Drawing for the job (mm, zero at the part's lowest x, y, z). Coordinates: 2 decimals unless noted, no trailing zeros. Order: outer loops, then holes, each group sorted by start corner. A loop starts at its lowest first (then second) coordinate and runs counter-clockwise, first axis right, second up. Notation, with made-up numbers: (65, 86.25) - (113, 86.25) arc R8 cw to (113, 90.25) - close; hole circle Ø4 at (-20.75, 70.5). An arc over 180 degrees is marked (long way). Put each result on its own line as item: value. Start each with the question number.
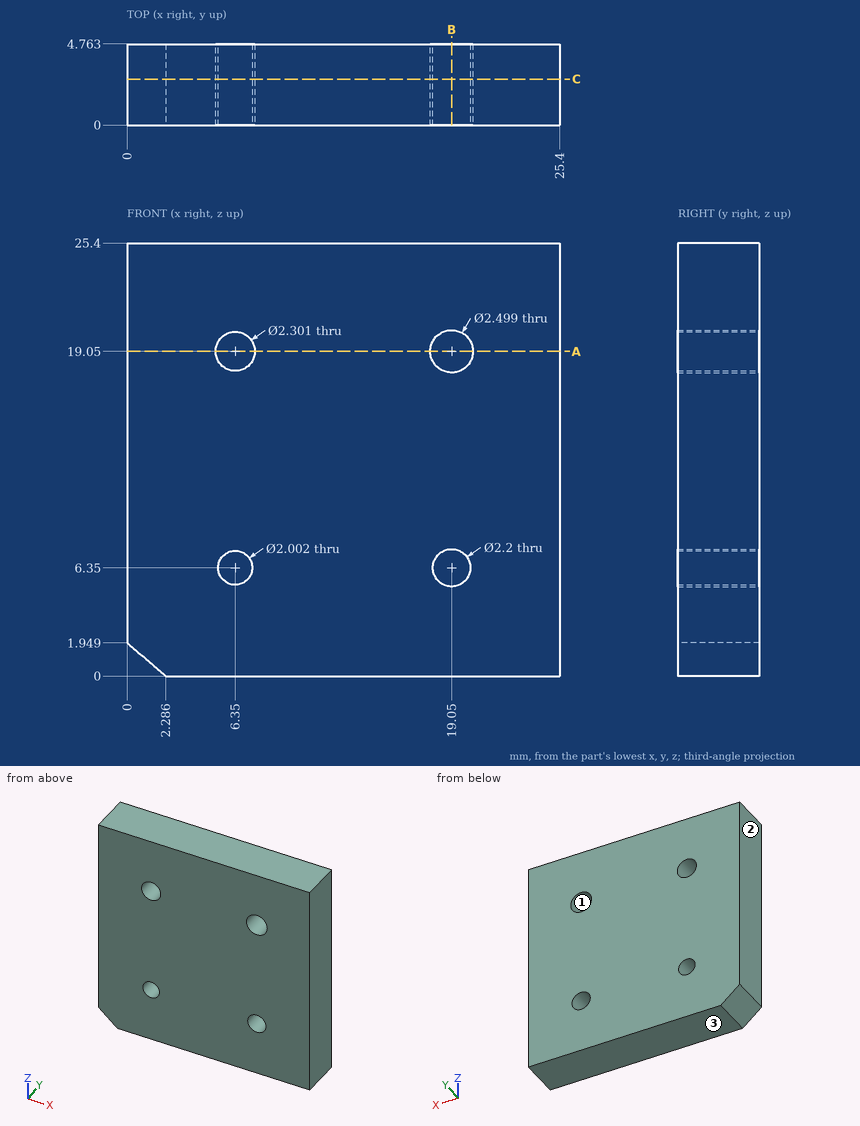
Item 1: Slice it at A-A, the plane z = 19.05. Give the cut face in (x, y).
Item 2: Slice it at C-C, the plane y = 2.7. Give the number of separate pieces and of enclosed holes in the cut face, plus the area to 3 significant figures.
Item 3: Pull direction Z, two halves, no side cores. Call the marked faces 1, 2 and 3: pulls with the +Z half, pulls with the -Z half, needs draft (parallel to the pull), parting line crosses it, or undercut.
Item 4: Wall check: line 1 along X through (y, z) = (1.15, 19.05); line 2 along X through (y, z) = (1.3, 6.35); line 3 along Z through (x, y) = (6.35, 2.7). Give the ranges that are in metal, low to high.
Item 5: Slice it at B-B, the plane x = 19.05. Give the cut face in (y, z).
Here are the results:
1. outline: (0, 0) - (5.2, 0) - (5.2, 4.76) - (0, 4.76) - close; (7.5, 0) - (17.8, 0) - (17.8, 4.76) - (7.5, 4.76) - close; (20.3, 0) - (25.4, 0) - (25.4, 4.76) - (20.3, 4.76) - close
2. separate pieces: 1
2. enclosed holes: 4
2. area: 627 mm^2
3. face 1: undercut
3. face 2: needs draft
3. face 3: pulls with the -Z half
4. line 1: x = 0 to 5.2, 7.5 to 17.8, 20.3 to 25.4
4. line 2: x = 0 to 5.35, 7.35 to 17.95, 20.15 to 25.4
4. line 3: z = 0 to 5.35, 7.35 to 17.9, 20.2 to 25.4
5. outline: (0, 0) - (4.76, 0) - (4.76, 5.25) - (0, 5.25) - close; (0, 7.45) - (4.76, 7.45) - (4.76, 17.8) - (0, 17.8) - close; (0, 20.3) - (4.76, 20.3) - (4.76, 25.4) - (0, 25.4) - close
